The model under review builds one solid part; all positions refer to its coordinate system, in mm. A direction names the side the tool comes from. Coordinates: 2 decimals unless noted, no trailing zeros. Write each loop counter-clockwise with the first axis right and the second up, starting at its lowest first coordinate (ties: lowest second). Pieces come first, ordered by that corner, then holes.
```python
from build123d import *

# Parameters (mm, degrees)
EXTRUDE_1_DEPTH              = 14.5
HOLE_START                   = -15
HOLE_WIZARD_M2_1_OUTLINE_R   = 1.9
HOLE_WIZARD_M2_1_DEPTH       = 1
HOLE_START_2                 = -14
HOLE_WIZARD_M2_1_2_OUTLINE_R = 1.05
HOLE_WIZARD_M2_1_2_DEPTH     = 1
SKETCH_5_R                   = 6
EXTRUDE_2_DEPTH              = 2.5
SKETCH_6_R                   = 3.5
EXTRUDE_3_DEPTH              = 2
CHAMFER_1_SIZE               = 0.5
CUT_EXTRUDE_1_REACH          = 27.323
SKETCH_7_R                   = 0.925
FILLET_1_R                   = 4
FILLET_2_R                   = 1
CUT_EXTRUDE_2_REACH          = 26.439
SKETCH_8_W                   = 8
SKETCH_8_H                   = 2
FILLET_3_R                   = 1


# Read off the part's stored shape, not the designer's step: M2 丸平ねじ用座ぐり穴1
with BuildPart() as part:
    # ｽｹｯﾁ1 → ﾎﾞｽ - 押し出し1 (new, symmetric)
    with BuildSketch(Plane(origin=(0, 0, 0), x_dir=(0, 0, -1), z_dir=(1, 0, 0))):
        Polygon((-15, -5), (15, -5), (15, 5), (13, 5), (13, -2.5), (-13, -2.5), (-13, 5), (-15, 5), align=None)
    extrude(amount=EXTRUDE_1_DEPTH, both=True)

    # M2 丸平ねじ用座ぐり穴1 outline → M2 丸平ねじ用座ぐり穴1 (cut)
    with BuildSketch(Plane.XY.offset(HOLE_START)):
        with Locations((-10.5, 1)):
            Circle(HOLE_WIZARD_M2_1_OUTLINE_R)
        with Locations((10.5, 1)):
            Circle(HOLE_WIZARD_M2_1_OUTLINE_R)
    hole_wizard_m2_1 = extrude(amount=HOLE_WIZARD_M2_1_DEPTH, mode=Mode.SUBTRACT)

    # Hole Wizard M2 _1 2 outline → Hole Wizard M2 _1 2 (cut)
    with BuildSketch(Plane.XY.offset(HOLE_START_2)):
        with Locations((-10.5, 1)):
            Circle(HOLE_WIZARD_M2_1_2_OUTLINE_R)
        with Locations((10.5, 1)):
            Circle(HOLE_WIZARD_M2_1_2_OUTLINE_R)
    hole_wizard_m2_1_2 = extrude(amount=HOLE_WIZARD_M2_1_2_DEPTH, mode=Mode.SUBTRACT)

    # ｽｹｯﾁ5 → ﾎﾞｽ - 押し出し2 (add)
    with BuildSketch(Plane.XZ.offset(5)):
        with Locations((-10.5, 0)):
            Circle(SKETCH_5_R)
    extrude(amount=-EXTRUDE_2_DEPTH)

    # ｽｹｯﾁ6 → ﾎﾞｽ - 押し出し3 (add)
    with BuildSketch(Plane.XZ.offset(5)):
        with Locations(Location((-10.5, 0, 0), (0, 0, 90))):
            Circle(SKETCH_6_R)
    extrude(amount=EXTRUDE_3_DEPTH)

    # 面取り1
    chamfer_1_edges = [part.edges().sort_by_distance(p)[0] for p in [
        (-10.5, -7, -3.5),
    ]]
    chamfer(chamfer_1_edges, length=CHAMFER_1_SIZE)

    # ｽｹｯﾁ7 → ｶｯﾄ - 押し出し1 (cut, up to next)
    with BuildSketch(Plane.XZ.offset(7), mode=Mode.PRIVATE) as cut_extrude_1_sk1:
        with Locations(Location((-10.5, 0, 0), (0, 0, 270))):
            Circle(SKETCH_7_R)
    cut_extrude_1_tool1 = extrude(cut_extrude_1_sk1.sketch, amount=-CUT_EXTRUDE_1_REACH, mode=Mode.PRIVATE) & part.part
    add(cut_extrude_1_tool1.solids().sort_by_distance((-10.5, -7, 0))[0], mode=Mode.SUBTRACT)

    # ﾌｨﾚｯﾄ1
    fillet_1_edges = [part.edges().sort_by_distance(p)[0] for p in [
        (-14.5, 5, 14),
        (14.5, 5, -14),
        (14.5, 5, 14),
        (-14.5, 5, -14),
    ]]
    fillet(fillet_1_edges, radius=FILLET_1_R)

    # ﾌｨﾚｯﾄ2
    fillet_2_edges = [part.edges().sort_by_distance(p)[0] for p in [
        (0, -5, -15),
        (0, -5, 15),
        (-14.5, -3.75, -4.472135955),
        (-14.5, -3.75, 4.472135955),
    ]]
    fillet(fillet_2_edges, radius=FILLET_2_R)

    # ｽｹｯﾁ8 → ｶｯﾄ - 押し出し2 (cut, up to next)
    with BuildSketch(Plane.XZ.offset(5), mode=Mode.PRIVATE) as cut_extrude_2_sk1:
        with Locations((0, -10)):
            Rectangle(SKETCH_8_W, SKETCH_8_H)
    cut_extrude_2_tool1 = extrude(cut_extrude_2_sk1.sketch, amount=-CUT_EXTRUDE_2_REACH, mode=Mode.PRIVATE) & part.part
    add(cut_extrude_2_tool1.solids().sort_by_distance((0, -5, -10))[0], mode=Mode.SUBTRACT)

    # ﾌｨﾚｯﾄ3
    fillet_3_edges = [part.edges().sort_by_distance(p)[0] for p in [
        (4, -3.75, -9),
        (-4, -3.75, -9),
        (-4, -3.75, -11),
        (4, -3.75, -11),
    ]]
    fillet(fillet_3_edges, radius=FILLET_3_R - 0.0001)  # a hair under: the kernel refuses the full size

    # ﾐﾗｰ1: M2 丸平ねじ用座ぐり穴1, Hole Wizard M2 _1 2 across plane
    add(hole_wizard_m2_1.mirror(Plane.XY), mode=Mode.SUBTRACT)
    add(hole_wizard_m2_1_2.mirror(Plane.XY), mode=Mode.SUBTRACT)


solid = part.part
```
Item 1: Take a section at D-D, the plane y = -5.5. Write out the cut boundary in (x, z) (3 decimals).
Solved:
outline: circle Ø7 at (-10.5, 0); hole circle Ø1.85 at (-10.5, 0)
Item 2: Machinability: for faces 5 (the face through (-8.745, 0.272, 14.507)), 6 (the face through (-3.699, -3.732, -9.285)), 7 (the face through (-14.5, -3, 11)), 8 (the face through (12, 1, -14)), which of the approach directions +Z, -Z, +X, -X, +Y, -Y give a long, thin tool a straight path to every point of the face, cutting with its end or side? Answer none if there is none.
Solved:
face 5: +Z
face 6: +Y, -Y
face 7: +Z, -X, +Y, -Y
face 8: -Z
Item 3: To check wall thickness, follow line 1 along Z through (x, y) = (-11, -1); line 2 along Y through (x, z) = (10.5, -13.25); line 3 along Y through (x, z) = (-10.5, 14.55). State the ranges of each line that lie inside material, in increasing order.
Solved:
line 1: z = -15 to -13, 13 to 15
line 2: y = -5 to -0.05, 2.05 to 5
line 3: y = -4.84 to -0.9, 2.9 to 5
Item 4: Mouldability with a two-part tool opening along Z and no side actions: class faces 1 (the face through (3.715, -3.732, -9.301)), 2 (the face through (-10, -7, -1)), 3 (the face through (-0.203, -4.699, 14.715)), 4 (the face through (3.699, -3.732, -10.715)) as pulls with the +Z half, pulls with the -Z half, needs draft (parallel to the pull), parting line crosses it, or undercut.
Solved:
face 1: undercut
face 2: needs draft
face 3: pulls with the +Z half
face 4: undercut
Item 5: Take a section at C-C, the plane z = 0. Write out the cut boundary in (x, y) (3 decimals), plus the area to 3 significant figures.
Solved:
outline: (-16.5, -5) - (-14, -5) - (-14, -6.5) - (-13.5, -7) - (-11.425, -7) - (-11.425, -2.5) - (-16.5, -2.5) - close; (-9.575, -7) - (-7.5, -7) - (-7, -6.5) - (-7, -5) - (14.5, -5) - (14.5, -2.5) - (-9.575, -2.5) - close
area: 82.9 mm2
Item 6: Take a section at B-B, the plane x = 1. Write out the cut boundary in (y, z).
Solved:
outline: (-5, -14) arc R1 ccw to (-4, -15) - (5, -15) - (5, -13) - (-2.5, -13) - (-2.5, -11) - (-5, -11) - close; (-5, -9) - (-2.5, -9) - (-2.5, 13) - (5, 13) - (5, 15) - (-4, 15) arc R1 ccw to (-5, 14) - close
Item 7: Take a section at A-A, the plane y = -1.75. Write out the cut boundary in (x, z), plus the area to 3 significant figures.
Solved:
outline: (-14.5, -15) - (14.5, -15) - (14.5, -13) - (-14.5, -13) - close; (-14.5, 13) - (14.5, 13) - (14.5, 15) - (-14.5, 15) - close
area: 116 mm2
Item 8: For pin 1 (1 mm diameter, centred on x = 8, z = -4, fed in from -Y); pin 2 (1.9 mm diameter, centred on x = 11, y = 1, fed in from -Z); pin 3 (1.5 mm diameter, centred on y = 0, z = 5, fed in from +X); pin 4 (3.5 mm diameter, centred on x = -10.5, y = 1, fed in from +Z), all flat-tipped, find the tip position at first contact; note any pin that passes through.
Solved:
pin 1: stops at y = -5
pin 2: stops at z = -14
pin 3: passes through
pin 4: stops at z = 14
